from build123d import *

# Parameters (mm, degrees)
BOSS_EXTRUDE1_DEPTH                      = 10
BOSS_EXTRUDE1_DEPTH_BACK                 = 10
SKETCH1_W                                = 22
SKETCH1_H                                = 35
CUT_EXTRUDE1_DEPTH                       = 30.837057496
CUT_EXTRUDE1_DEPTH_BACK                  = 30.837057496
SKETCH2_W                                = 12.4
SKETCH2_H                                = 10.2
CUT_EXTRUDE2_DEPTH                       = 5.2
MIRROR1_AT_THE_SECOND_PLANE_COPY_1_DEPTH = 5.2


with BuildPart() as part:
    # Sketch1 → Boss-Extrude1 (new, two sides: drawn at the far end of the back side and taken through both)
    with BuildSketch(Plane(origin=(0, 0, 0), x_dir=(0, 0, -1), z_dir=(1, 0, 0)).offset(-BOSS_EXTRUDE1_DEPTH_BACK)):
        Rectangle(SKETCH1_W, SKETCH1_H)
    extrude(amount=BOSS_EXTRUDE1_DEPTH + BOSS_EXTRUDE1_DEPTH_BACK)

    # Sketch2 → Cut-Extrude1 (cut, two sides: drawn at the far end of the back side and taken through both)
    with BuildSketch(Plane.XY.offset(11).offset(-CUT_EXTRUDE1_DEPTH_BACK)):
        Rectangle(SKETCH2_W, SKETCH2_H)
    extrude(amount=CUT_EXTRUDE1_DEPTH + CUT_EXTRUDE1_DEPTH_BACK, mode=Mode.SUBTRACT)

    # Sketch3 → Cut-Extrude2 (cut)
    with BuildSketch(Plane(origin=(0, 17.5, 0), x_dir=(1, 0, 0), z_dir=(0, 1, 0))):
        Polygon((3.6, 7.578460969), (0, 9.656921938), (-3.6, 7.578460969), (-3.6, 3.421539031), (0, 1.343078062), (3.6, 3.421539031), align=None)
    cut_extrude2 = extrude(amount=-CUT_EXTRUDE2_DEPTH, mode=Mode.SUBTRACT)

    # Mirror1: Cut-Extrude2 across plane
    add(cut_extrude2.mirror(Plane.ZX), mode=Mode.SUBTRACT)

    # Mirror1 at the second plane: Cut-Extrude2 across plane
    add(cut_extrude2.mirror(Plane.XY), mode=Mode.SUBTRACT)

    # Mirror1 at the second plane copy 1 sketc → Mirror1 at the second plane copy 1 (cut)
    with BuildSketch(Plane.XZ.offset(17.5)):
        Polygon((3.6, 7.578460969), (0, 9.656921938), (-3.6, 7.578460969), (-3.6, 3.421539031), (0, 1.343078062), (3.6, 3.421539031), align=None)
    extrude(amount=-MIRROR1_AT_THE_SECOND_PLANE_COPY_1_DEPTH, mode=Mode.SUBTRACT)


solid = part.part
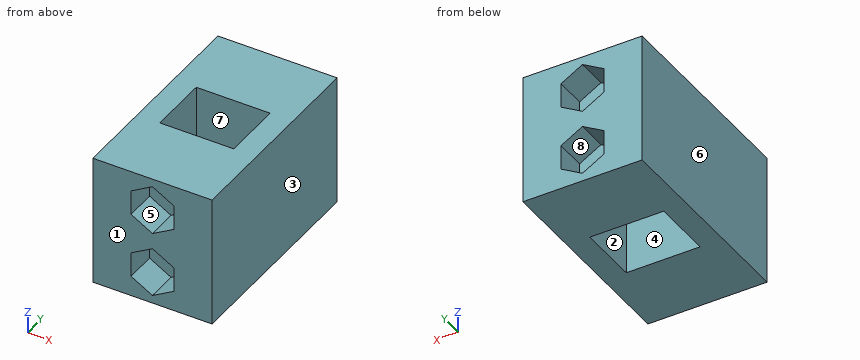
Build history of the part. All positions in model axes, mm. Face numbers are marked on the shaded views. A direction names the side the tool comes from. Round coordinates to 2 decimals unless told otherwise and drop trailing zeros. Write each loop counter-clockwise with the first axis right and the second up, starting at its lowest first coordinate (ties: lowest second). Pieces come first, ordered by that corner, then holes. Notation, with made-up numbers: M -20.75,29 L 22.25,29 A28 cw 22.25,58 Z; hole C 62.5,35 d4. An arc over 180 degrees is marked long. Answer in a Markdown table with one row per item.
1. Saw through at C-C (z = 4.75). List the corners of the cut face in (x, y).
Geometry check:
| item | result |
|---|---|
| outline | M -10,-17.5 L -3.6,-17.5 L -3.6,-12.3 L 3.6,-12.3 L 3.6,-17.5 L 10,-17.5 L 10,17.5 L 3.6,17.5 L 3.6,12.3 L -3.6,12.3 L -3.6,17.5 L -10,17.5 Z; hole M -6.2,-5.1 L 6.2,-5.1 L 6.2,5.1 L -6.2,5.1 Z |
2. Which spindle directions (+Z, -Z, +X, -X, +Y, -Y) get a long thin tool onto all of the face, cutting with end or side? Do the marked faces 5, 6, 7 and 8. Say none if no direction does.
Geometry check:
| item | result |
|---|---|
| face 5 | -Y |
| face 6 | +Z, -Z, -X, +Y, -Y |
| face 7 | +Z, -Z |
| face 8 | +Y |
3. Saw through at B-B (x = 5.25). List the corners of the cut face in (y, z), and give its area (3 significant figures).
Geometry check:
| item | result |
|---|---|
| outline | M -17.5,-11 L -5.1,-11 L -5.1,11 L -17.5,11 Z; M 5.1,-11 L 17.5,-11 L 17.5,11 L 5.1,11 Z |
| area | 546 mm2 |
4. Probe L1, parallel to Y at x = -4.75, z = 4.5; L2, parallel to X at y = 4.5, z = 3.75; L3, parallel to Y at x = -3.25, z = 7. List the from-to ranges inside material, lowest first. Write a range as [from, to].
Geometry check:
| item | result |
|---|---|
| L1 | [-17.5, -5.1], [5.1, 17.5] |
| L2 | [-10, -6.2], [6.2, 10] |
| L3 | [-12.3, -5.1], [5.1, 12.3] |
5. Flat gauge pins, fed straight in: P1, Ø3.5, axis at x = -0.5, z = -5, coming from the -Y side; P2, Ø2, axis at x = -0.5, z = 6.5, coming from the +Y side. Where does each tip first touch, or does it go through?
Geometry check:
| item | result |
|---|---|
| P1 | y = -12.3 |
| P2 | y = 12.3 |
6. Mould opens along Y. For the marked faces 1, 2, 3 and 4 say: +Y half, -Y half, draft (parallel to the pull), parting line (faces both ways), or undercut.
Geometry check:
| item | result |
|---|---|
| face 1 | -Y half |
| face 2 | undercut |
| face 3 | draft |
| face 4 | undercut |
7. Saw through at D-D (x = -1.25). List the corners of the cut face in (y, z), and give its area (3 significant figures).
Geometry check:
| item | result |
|---|---|
| outline | M -17.5,-11 L -5.1,-11 L -5.1,11 L -17.5,11 L -17.5,8.94 L -12.3,8.94 L -12.3,2.06 L -17.5,2.06 L -17.5,-2.06 L -12.3,-2.06 L -12.3,-8.94 L -17.5,-8.94 Z; M 5.1,-11 L 17.5,-11 L 17.5,-8.94 L 12.3,-8.94 L 12.3,-2.06 L 17.5,-2.06 L 17.5,2.06 L 12.3,2.06 L 12.3,8.94 L 17.5,8.94 L 17.5,11 L 5.1,11 Z |
| area | 403 mm2 |
8. Saw through at A-A (y = -14). List the corners of the cut face in (x, z).
Geometry check:
| item | result |
|---|---|
| outline | M -10,-11 L 10,-11 L 10,11 L -10,11 Z; hole M -3.6,-7.58 L 0,-9.66 L 3.6,-7.58 L 3.6,-3.42 L 0,-1.34 L -3.6,-3.42 Z; hole M -3.6,3.42 L 0,1.34 L 3.6,3.42 L 3.6,7.58 L 0,9.66 L -3.6,7.58 Z |
